Input: dimensioned drawing with shaded views. Units: mm. Origin: part minimum x, y, z. A direction names the side the tool comes from. Round coordinates to 2 decimals unless told otherwise and drop trailing zeros. Loops run counter-clockwise (first coordinate to the right, second up) from the corner with the lowest first, then second, coordinate; pieces in that order, holes last. Notation, with made-up numbers: M -16.75,75.5 L 42.25,75.5 A17 cw 42.25,91.5 Z; hole C 82,87.5 d2. An arc over 180 degrees is marked long. One line per item, written item: value.
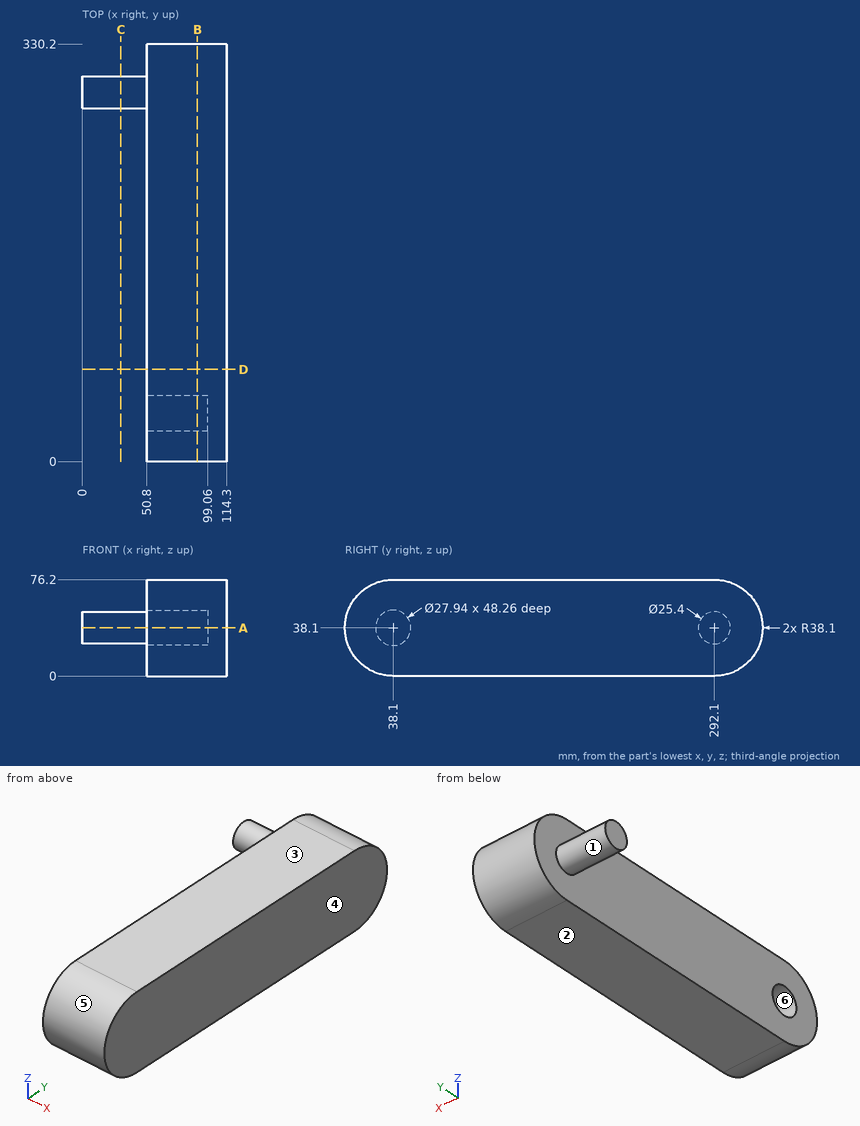
1. Section query C-C (x = 30.5). Return the cut outline in (y, z), and give its area (3 significant figures).
Report:
outline: C 292.1,38.1 d25.4
area: 507 mm2
2. Ray query, line 1 (Z direction, x = 83, y = 38.1); line 2 (Y direction, x = 75.5, z = 38.1); line 3 (X direction, y = 58, z = 21). Return the intervals inside material, ascending. Write a range as [from, to].
Report:
line 1: z = [0, 24.13], [52.07, 76.2]
line 2: y = [0, 24.13], [52.07, 330.2]
line 3: x = [50.8, 114.3]
3. Reachability of the marked faces 1 and 2 from +Z, -Z, +X, -X, +Y, -Y: full face, straight path, thin tool, end or side. Return the list, or none.
Report:
face 1: -X
face 2: -Z, +X, -X, +Y, -Y
4. Pin query (flat end, axial travel): pin 1 (12 mm diameter, centred on x = 97.5, z = 18.5, fed in from +Y); pin 2 (14 mm diameter, centred on y = 35.5, z = 36.5, fed in from -X); pin 3 (1.5 mm diameter, centred on x = 84, z = 46.5, fed in from +Y). Return the tip coordinate at first contact, or that it passes through.
Report:
pin 1: stops at y = 327.69
pin 2: stops at x = 99.06
pin 3: stops at y = 329.42
5. Pull-direction query (Z, two-part tool) for the marked faces 3, 4, 5 and 6; classes: released by +Z, released by -Z, zero draft, split by the parting line, or undercut.
Report:
face 3: released by +Z
face 4: zero draft
face 5: split by the parting line
face 6: undercut
6. Section query D-D (y = 73). Return the cut outline in (x, z).
Report:
outline: M 50.8,0 L 114.3,0 L 114.3,76.2 L 50.8,76.2 Z
7. Section query B-B (x = 91). Return the cut outline in (y, z).
Report:
outline: M 38.1,0 L 292.1,0 A38.1 ccw 292.1,76.2 L 38.1,76.2 A38.1 ccw Z; hole C 38.1,38.1 d27.94
8. Section query A-A (z = 38.1). Return the cut outline in (x, y).
Report:
outline: M 0,279.4 L 50.8,279.4 L 50.8,52.07 L 99.06,52.07 L 99.06,24.13 L 50.8,24.13 L 50.8,0 L 114.3,0 L 114.3,330.2 L 50.8,330.2 L 50.8,304.8 L 0,304.8 Z
